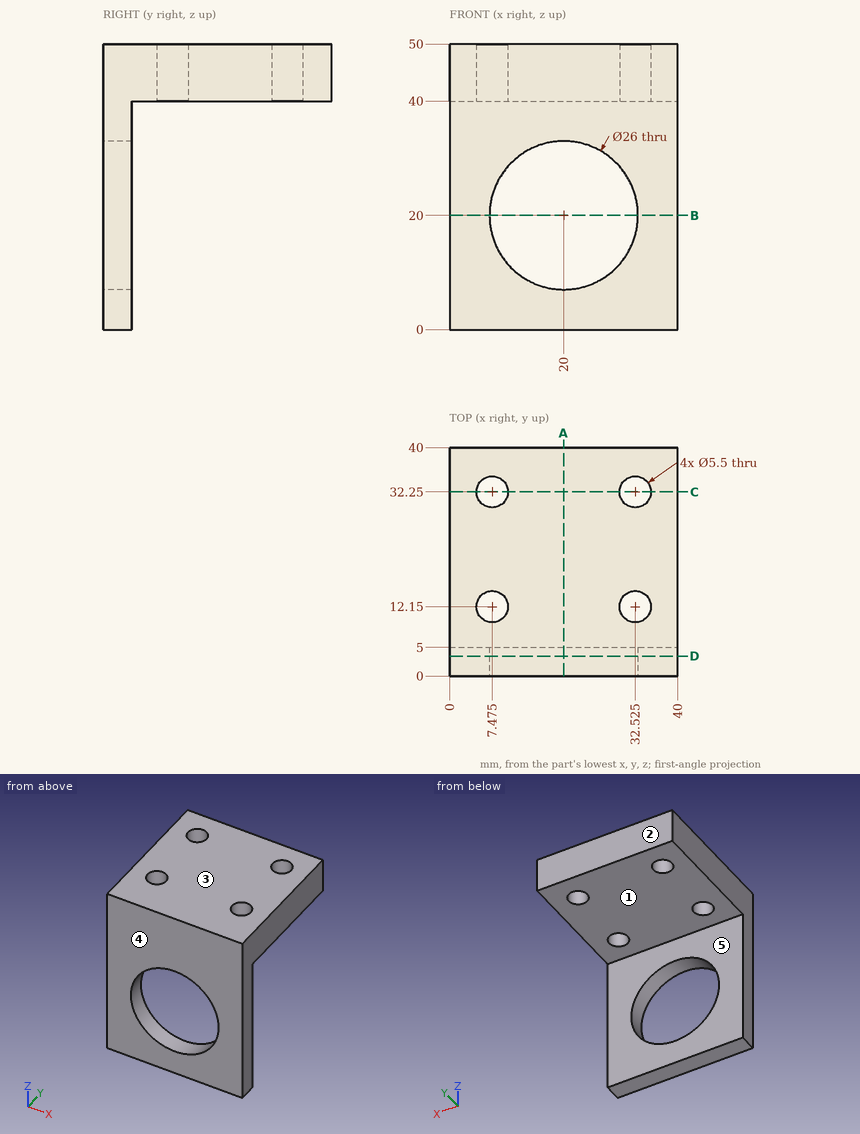
The drawing under review shows one solid part. Ordinate dimensions are in mm from its lowest x, y, z. A direction names the side the tool comes from. Coordinates: 2 decimals unless noted, no trailing zeros. Write each loop counter-clockwise with the first axis right and the second up, starting at its lowest first coordinate (ties: lowest second). Pieces come first, ordered by that corner, then holes. Notation, with made-up numbers: (12, 17) - (37, 17) arc R30 cw to (37, 41) - close; hole circle Ø1 at (11.5, 33). An arc over 180 degrees is marked (long way). Answer as CSV lines item,"result".
(1) Mouldability with a two-part tool opening along Y and no side actions: class the marked faces 3, 4 and 5 as pulls with the +Y half, pulls with the -Y half, needs draft (parallel to the pull), parting line crosses it, or undercut.
Data:
face 3,"needs draft"
face 4,"pulls with the -Y half"
face 5,"pulls with the +Y half"
(2) Tool access review of the marked faces 1 and 2: name each direction out of +Z, -Z, +X, -X, +Y, -Y from which nothing blocks a thin tool from reaching the whole face with its end or side.
Data:
face 1,"-Z, +X, -X, +Y"
face 2,"+Z, -Z, +X, -X, +Y"
(3) Clearance check with flat-ended pins moving along their axes: pin 1 Ø5 at (x, y) = (32.525, 32.25) entering from +Z; pin 2 Ø12 at (x, z) = (27.5, 25.5) entering from +Y; pin 3 Ø3 at (x, y) = (8, 4.5) entering from -Z. State where each tip first meets the part, or that it passes through.
Data:
pin 1,"passes through"
pin 2,"stops at y = 5"
pin 3,"stops at z = 0"
(4) We need section A-A (x = 20). Give the boundary of the cut face in (y, z).
Data:
outline,"(0, 0) - (5, 0) - (5, 7) - (0, 7) - close; (0, 33) - (5, 33) - (5, 40) - (40, 40) - (40, 50) - (0, 50) - close"
(5) We need section B-B (z = 20). Give the boundary of the cut face in (x, y).
Data:
outline,"(0, 0) - (7, 0) - (7, 5) - (0, 5) - close; (33, 0) - (40, 0) - (40, 5) - (33, 5) - close"
(6) We need section D-D (y = 3.5). Give the boundary of the cut face in (x, z), plus the area to 3 significant figures.
Data:
outline,"(0, 0) - (40, 0) - (40, 50) - (0, 50) - close; hole circle Ø26 at (20, 20)"
area,"1,470 mm2"
(7) We need section C-C (y = 32.25). Give the boundary of the cut face in (x, z) (3 decimals).
Data:
outline,"(0, 40) - (4.725, 40) - (4.725, 50) - (0, 50) - close; (10.225, 40) - (29.775, 40) - (29.775, 50) - (10.225, 50) - close; (35.275, 40) - (40, 40) - (40, 50) - (35.275, 50) - close"
(8) For line 1 along X through (y, z) = (12.15, 45.25) (3 decimals); line 2 along Y through (x, z) = (10, 42); line 3 along Z through (x, y) = (26.5, 7), list the stretches that pass through material, from the lowest coordinate up. Write a range as [from, to].
Data:
line 1,"x = [0, 4.725], [10.225, 29.775], [35.275, 40]"
line 2,"y = [0, 11.06], [13.24, 31.16], [33.34, 40]"
line 3,"z = [40, 50]"
